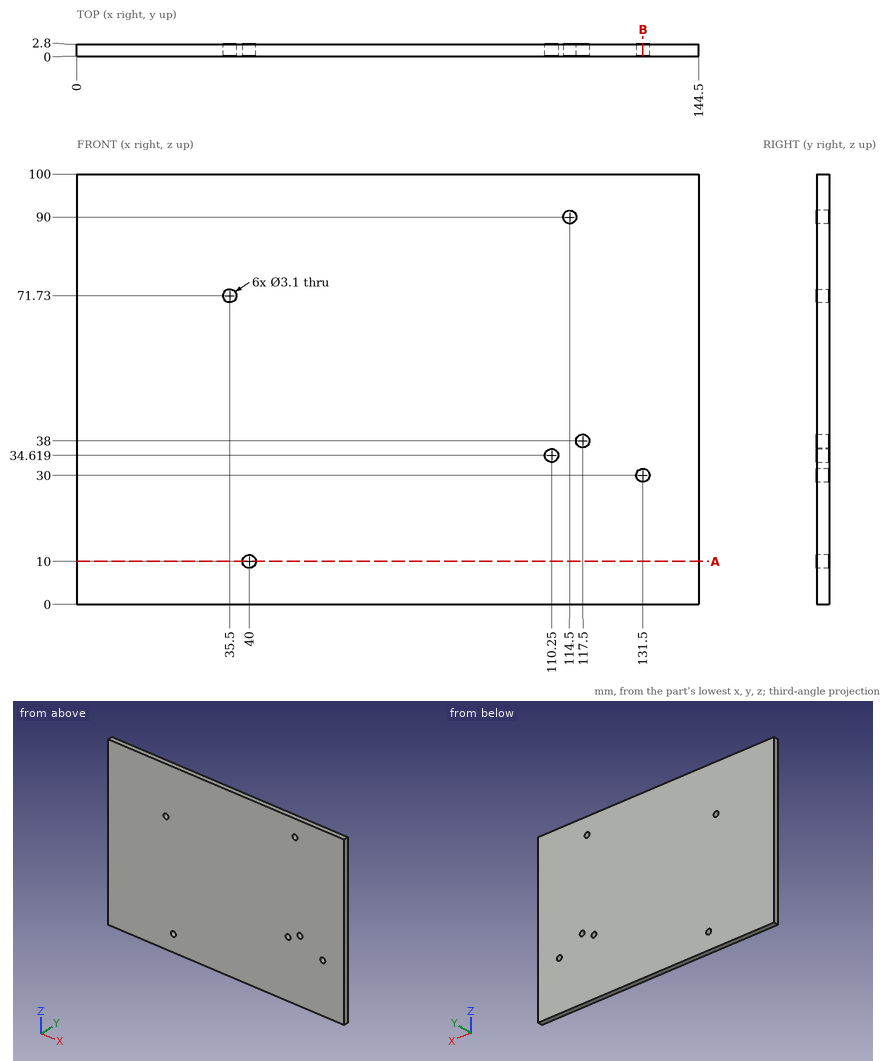
Verification items for this drawing (mm, ordinates from the low corner). Give positions to 0.01 mm unless a question says otherwise; leave off trailing zeros. Write each loop counter-clockwise with the first axis right and the second up, starting at its lowest first coordinate (ties: lowest second). Pieces come first, ordered by that corner, then holes.
1) Section check A-A, the plane z = 10. Record the boundary of the cut face in (x, y), and give its area (3 significant figures).
2) Section check B-B, the plane x = 131.5. Record the boundary of the cut face in (y, z).
3) Material ranges on L1, parallel to Z at x = 114.5, y = 1.6; L2, parallel to X at y = 0.9, z = 10; L3, parallel to X at y = 2.05, z = 71.73, recorded low to high.
Computed:
1. outline: (0, 0) - (38.45, 0) - (38.45, 2.8) - (0, 2.8) - close; (41.55, 0) - (144.5, 0) - (144.5, 2.8) - (41.55, 2.8) - close
1. area: 396 mm2
2. outline: (0, 0) - (2.8, 0) - (2.8, 28.45) - (0, 28.45) - close; (0, 31.55) - (2.8, 31.55) - (2.8, 100) - (0, 100) - close
3. L1: z = 0 to 88.45, 91.55 to 100
3. L2: x = 0 to 38.45, 41.55 to 144.5
3. L3: x = 0 to 33.95, 37.05 to 144.5
